```python
from build123d import *

# Parameters (mm, degrees)
F0_R     = 1.85
F1_DEPTH = 2.5


with BuildPart() as f1:
    # F0 (on Front) → F1 (new body, symmetric)
    with BuildSketch(Plane.XZ):
        with BuildLine():
            Line((-56.121855, 29.058371), (-7.998775, 0.139999))
            ThreePointArc((-7.998775, 0.139999), (0, -8), (7.998775, 0.139999))
            Line((7.998775, 0.139999), (56.121855, 29.058371))
            ThreePointArc((56.121855, 29.058371), (67.708993, 38.193603), (53.071797, 40.055513))
            Line((53.071797, 40.055513), (-53.071797, 40.055513))
            ThreePointArc((-53.071797, 40.055513), (-67.708993, 38.193603), (-56.121855, 29.058371))
        make_face()
        Circle(F0_R, mode=Mode.SUBTRACT)
        with Locations((-60, 36.055513)):
            Circle(F0_R, mode=Mode.SUBTRACT)
        with BuildLine():
            Line((-45.577795, 32.055513), (45.577795, 32.055513))
            Line((45.577795, 32.055513), (3.878145, 6.997142))
            ThreePointArc((3.878145, 6.997142), (0, 8), (-3.878145, 6.997142))
            Line((-3.878145, 6.997142), (-45.577795, 32.055513))
        make_face(mode=Mode.SUBTRACT)
        with Locations((60, 36.055513)):
            Circle(F0_R, mode=Mode.SUBTRACT)
    extrude(amount=F1_DEPTH, both=True)


solid = f1.part
```
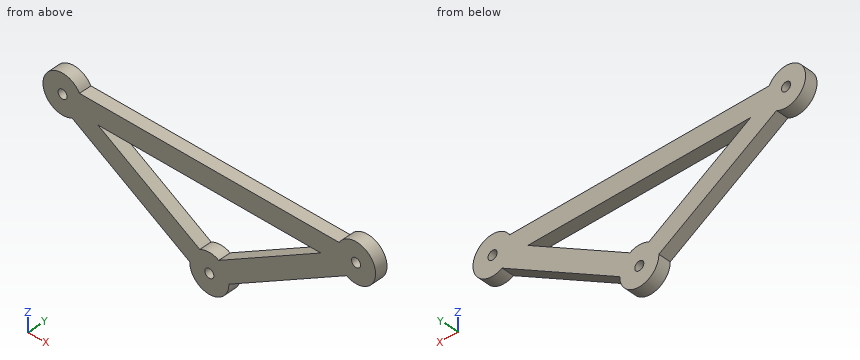
Here's how the part is built. I have some questions about the finished solid (model axes, mm). Give positions to 0.01 mm unless a question says otherwise; leave off trailing zeros. Loops run counter-clockwise (first coordinate to the right, second up) from the corner with the lowest first, then second, coordinate; pieces in that order, holes last. Notation, with made-up numbers: M -20,64 L 16,64 A25 cw 16,93 Z; hole C -27,65 d6. An arc over 180 degrees is marked long. Use one line per item in the form item = value. Start each with the question number.
Q1. If we section it at B-B (x = 0): Write out the boundary of the cut face in (y, z).
Q2. Will these pins go through, and if not, where does the flat tip stop? pin 1 Ø4 at (x, z) = (11.5, 15.5) entering from +Y; pin 2 Ø2.5 at (x, y) = (8.5, -1) entering from +Z; pin 3 Ø2.5 at (x, y) = (12, 0) entering from -Z.
Q3. If we section it at A-A (x = 60): Write out the boundary of the cut face in (y, z), then the cut area to 3 significant figures.
Q4. If we section it at C-C (y = -0.95): Write out the boundary of the cut face in (x, z), then the cut area to 3 significant figures.
Q5. I need wall thicknesses on line 1 along Z through (x, y) = (-60, -1.4); line 2 along Z through (x, y) = (-1, -1.65); line 3 along X through (y, z) = (-1.85, 35). Which ranges of each line are inside material? Lowest first, please.
Q6. If we section it at D-D (z = 17.5): Write out the boundary of the cut face in (x, y).
Taken from the geometry:
q1.outline = M -2.5,-8 L 2.5,-8 L 2.5,-1.85 L -2.5,-1.85 Z; M -2.5,1.85 L 2.5,1.85 L 2.5,8 L -2.5,8 Z; M -2.5,32.06 L 2.5,32.06 L 2.5,40.06 L -2.5,40.06 Z
q2.pin_1 = through
q2.pin_2 = 40.06
q2.pin_3 = 1.79
q3.outline = M -2.5,28.06 L 2.5,28.06 L 2.5,34.21 L -2.5,34.21 Z; M -2.5,37.91 L 2.5,37.91 L 2.5,44.06 L -2.5,44.06 Z
q3.area = 61.5 mm^2
q4.outline = M -56.12,29.06 L -8,0.14 A8 ccw long 8,0.14 L 56.12,29.06 A8 ccw long 53.07,40.06 L -53.07,40.06 A8 ccw long Z; hole C -60,36.06 d3.7; hole M -45.58,32.06 L -3.88,7 A8 cw 3.88,7 L 45.58,32.06 Z; hole C 0,0 d3.7; hole C 60,36.06 d3.7
q4.area = 2,260 mm^2
q5.line_1 = 28.06 to 34.21, 37.91 to 44.06
q5.line_2 = -7.94 to -1.56, 1.56 to 7.94, 32.06 to 40.06
q5.line_3 = -67.93 to -61.52, -58.48 to 58.48, 61.52 to 67.93
q6.outline = M -36.89,-2.5 L -21.36,-2.5 L -21.36,2.5 L -36.89,2.5 Z; M 21.36,-2.5 L 36.89,-2.5 L 36.89,2.5 L 21.36,2.5 Z
